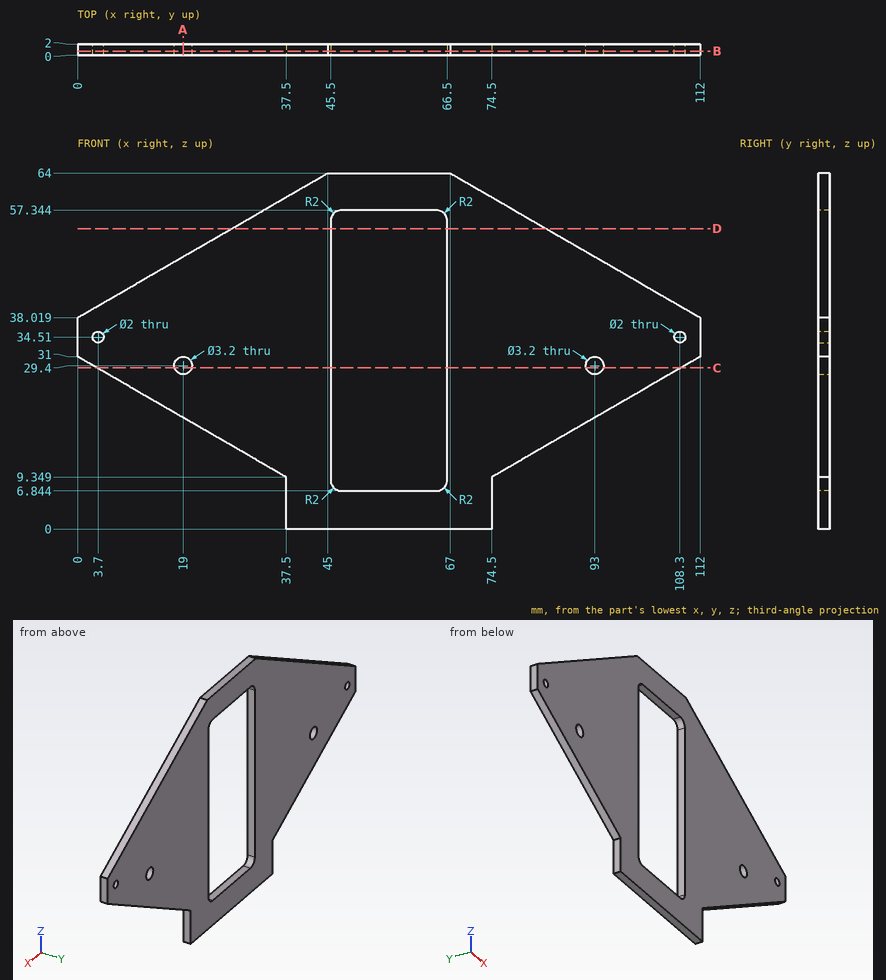
Design review of the part shown in the three views and the two pictorial views. Dimensions are in mm from the part's minimum x, y and z. Coordinates: 2 decimals unless noted, no trailing zeros. Order: outer loops, then holes, each group sorted by start corner. A loop starts at its lowest first (then second) coordinate and runs counter-clockwise, first axis right, second up. Notation, with made-up numbers: (-15.75, 17) -> (16.25, 17) arc R12 cw to (16.25, 34) -> close; hole circle Ø11 at (47, 37). An arc over 180 degrees is marked (long way). Use one line per item in the form item = value. Start each with the question number.
(1) Add section A-A on x = 19. State the section outline as (y, z) points.
(2) For probe 1 along X at (y, z) = (0.75, 29.4); probe 2 along X at (y, z) = (1, 36.5); probe 3 along X at (y, z) = (0.6, 30.5) (1 decimal), list the stretches that pass through material, from the lowest coordinate up.
(3) Add section C-C on z = 29. State the section outline as (x, y) points.
(4) Add section B-B on y = 0.7. State the section outline as (x, z) points, plus the area to 3 significant figures.
(5) Insertion check: pin 1 (1 mm diameter, centred on y = 1.5, z = 4.5, fed in from -X); pin 2 (3 mm diameter, centred on x = 19, z = 29.4, fed in from +Y); pin 3 (1 mm diameter, centred on x = 88.5, y = 0.5, fed in from -Z); pin 4 (0.6 mm diameter, centred on y = 0.5, z = 43, fed in from -X) (1 decimal). Each pin has a flat end and moves straight along its axis. Give the tip position at first contact, or say it passes through.
(6) Add section D-D on z = 54. State the section outline as (x, y) points.
Answer block:
q1.outline = (0, 20.03) -> (2, 20.03) -> (2, 27.8) -> (0, 27.8) -> close; (0, 31) -> (2, 31) -> (2, 48.99) -> (0, 48.99) -> close
q2.probe_1 = 2.77 to 17.4, 20.6 to 45.5, 66.5 to 91.4, 94.6 to 109.23
q2.probe_2 = 0 to 45.5, 66.5 to 112
q2.probe_3 = 0.9 to 17.8, 20.2 to 45.5, 66.5 to 91.8, 94.2 to 111.1
q3.outline = (3.46, 0) -> (17.45, 0) -> (17.45, 2) -> (3.46, 2) -> close; (20.55, 0) -> (45.5, 0) -> (45.5, 2) -> (20.55, 2) -> close; (66.5, 0) -> (91.45, 0) -> (91.45, 2) -> (66.5, 2) -> close; (94.55, 0) -> (108.54, 0) -> (108.54, 2) -> (94.55, 2) -> close
q4.outline = (0, 31) -> (37.5, 9.35) -> (37.5, 0) -> (74.5, 0) -> (74.5, 9.35) -> (112, 31) -> (112, 38.02) -> (67, 64) -> (45, 64) -> (0, 38.02) -> close; hole circle Ø2 at (3.7, 34.51); hole circle Ø3.2 at (19, 29.4); hole (45.5, 8.84) arc R2 ccw to (47.5, 6.84) -> (64.5, 6.84) arc R2 ccw to (66.5, 8.84) -> (66.5, 55.34) arc R2 ccw to (64.5, 57.34) -> (47.5, 57.34) arc R2 ccw to (45.5, 55.34) -> close; hole circle Ø3.2 at (93, 29.4); hole circle Ø2 at (108.3, 34.51)
q4.area = 3,410 mm²
q5.pin_1 = 37.5
q5.pin_2 = through
q5.pin_3 = 17.14
q5.pin_4 = 8.1
q6.outline = (27.68, 0) -> (45.5, 0) -> (45.5, 2) -> (27.68, 2) -> close; (66.5, 0) -> (84.32, 0) -> (84.32, 2) -> (66.5, 2) -> close
